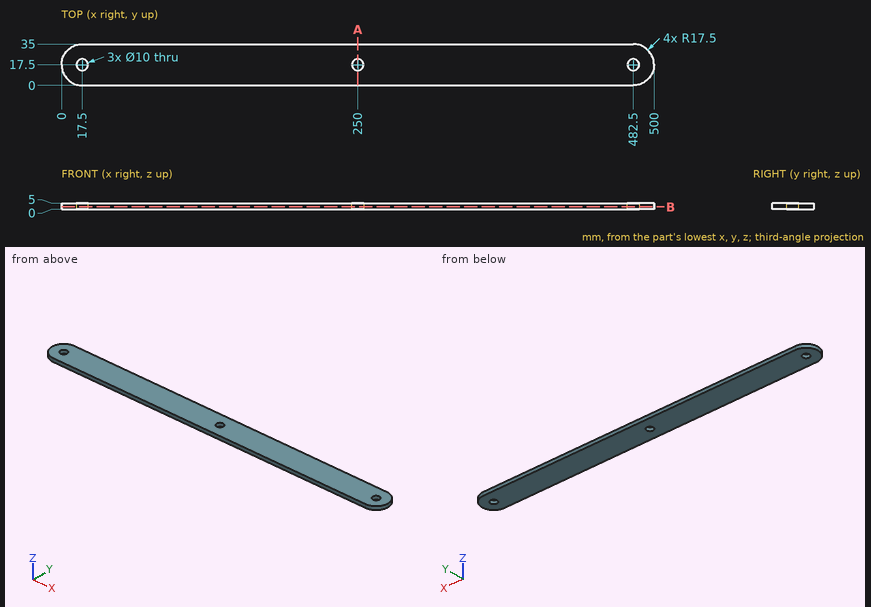
Check sheet for the drawn part. Datum: minimum x, y, z corner. Units: mm. Give positions to 0.01 mm unless a question says otherwise; leave off trailing zeros. Order: outer loops, then holes, each group sorted by start corner. A loop starts at its lowest first (then second) coordinate and runs counter-clockwise, first axis right, second up. Notation, with made-up numbers: (39, 47) - (93, 47) arc R32 cw to (93, 83) - close; hole circle Ø5 at (87.5, -34). An arc over 180 degrees is marked (long way). Answer in a Markdown table with one row per item. Add a question column.
Q1. Gauge pin test, flat end, axial feed: pin 1 (9 mm diameter, centred on x = 17.5, y = 17.5, fed in from -Z). Record the tip position at first contact, or that the pin passes through.
Q2. Cross-section at A-A, the plane x = 250. Enter the section's corners in (y, z).
Q3. Cross-section at B-B, the plane z = 2.2. Count the separate pieces of the cut face and the enclosed holes in it, then the cut area to 3 significant figures.
Q4. Material ranges on probe 1 along X at (y, z) = (18.5, 1.05); probe 2 along Y at (x, z) = (17.5, 2.45); probe 3 along X at (y, z) = (15, 2.5), recorded low to high. Write a range as from..to.
Check values:
| question | item | result |
|---|---|---|
| 1 | pin 1 | passes through |
| 2 | outline | (0, 0) - (12.5, 0) - (12.5, 5) - (0, 5) - close; (22.5, 0) - (35, 0) - (35, 5) - (22.5, 5) - close |
| 3 | separate pieces | 1 |
| 3 | enclosed holes | 3 |
| 3 | area | 17,000 mm^2 |
| 4 | probe 1 | x = 0.03..12.6, 22.4..245.1, 254.9..477.6, 487.4..499.97 |
| 4 | probe 2 | y = 0..12.5, 22.5..35 |
| 4 | probe 3 | x = 0.18..13.17, 21.83..245.67, 254.33..478.17, 486.83..499.82 |
